The listing builds one solid part. Answer for the finished solid, in the listing's coordinates (mm). A direction names the side the tool comes from. Give positions to 0.01 mm unless a question says otherwise; leave off trailing zeros. Write each loop counter-clockwise with the first axis right and the second up, starting at its lowest first coordinate (ties: lowest second). Pieces come first, ordered by that corner, then holes. Notation, with made-up numbers: (-20.5, 11) - (28.5, 11) arc R31 ccw to (28.5, 35) - close; hole circle Ø8 at (76.5, 62). An arc over 180 degrees is marked (long way). Write each question's results on one line, items separated by ' | '. Start each with the question number.
Q1. Flat-ended cylindrical pins translate along their axes: pin 1 Ø5 at (x, y) = (30.78, -3.04) entering from -Z; pin 2 Ø7 at (x, y) = (6, -4.5) entering from -Z. Find the tip coordinate at first contact, or state that the pin passes through.
Q2. Section C-C (z = -14) is taken. Determine the outline of the cut face in (x, y) (3 decimals).
Q3. Section D-D (x = 33.5) is taken. Determine the outline of the cut face in (y, z) (3 decimals), plus the area to 3 significant figures.
Q4. Section A-A (z = -8.5) is taken. Determine the outline of the cut face in (x, y), plus the area to 3 significant figures.
Q5. Section B-B (y = 1) is taken. Determine the outline of the cut face in (x, z).
Q6. Find the intervals of material crossed by probe 1 along X at (y, z) = (2.25, 9); probe 2 along Z at (x, y) = (7, 0); probe 3 along Z at (x, y) = (22.5, -8.5), in increasing order.
Q7. For a pull along X with two mould halves and no side action, classify faces 4 (the face through (11.43, 0, 2.5)), 5 (the face through (35.56, 0, 0)), 6 (the face through (10, -9.392, -1)) as pulls with the +X half, pulls with the -X half, needs draft (parallel to the pull), parting line crosses it, or undercut.
Q8. For faces 1 (the face through (18, 0, -19.473)), 2 (the face through (5, -3, -13.123)), 3 (the face through (18, 0, -13.123)), determine the directions among +Z, -Z, +X, -X, +Y, -Y from which every point of the face is accessible in a straight line to the end or side of a thin tool.
```python
from build123d import *

# Parameters (mm, degrees)
F0_W     = 19.05
F0_H     = 38.1
F0_R     = 3.175
F1_DEPTH = 35.56
F2_R     = 3.175
F3_DEPTH = 6.35
F4_W     = 12.7
F4_H     = 31.75
F5_DEPTH = 35.56


with BuildPart() as f1:
    # F0 (on Right) → F1 (new body)
    with BuildSketch(Plane.YZ):
        with Locations((0.13327, -0.423332)):
            Rectangle(F0_W, F0_H)
        with Locations((0.13327, 5.926668)):
            Circle(F0_R, mode=Mode.SUBTRACT)
    extrude(amount=F1_DEPTH)

    # F2 (on face) → F3 (cut)
    with BuildSketch(Plane(origin=(0, 0, -19.473332), x_dir=(1, 0, 0), z_dir=(0, 0, -1))):
        with Locations((4.7752, 3.04173)):
            Circle(F2_R)
        with Locations((30.7848, 3.04173)):
            Circle(F2_R)
    extrude(amount=-F3_DEPTH, mode=Mode.SUBTRACT)

    # F4 (on face) → F5 (cut)
    with BuildSketch(Plane.XZ.offset(9.39173)):
        with Locations((17.78, 2.751668)):
            Rectangle(F4_W, F4_H)
    extrude(amount=-F5_DEPTH, mode=Mode.SUBTRACT)


solid = f1.part
```
Answers below:
1) pin 1: stops at z = -13.12 | pin 2: stops at z = -19.47
2) outline: (0, -9.392) - (35.56, -9.392) - (35.56, 9.658) - (0, 9.658) - close; hole circle Ø6.35 at (4.775, -3.042); hole circle Ø6.35 at (30.785, -3.042)
3) outline: (-9.392, -19.473) - (-4.687, -19.473) - (-4.687, -13.123) - (-1.396, -13.123) - (-1.396, -19.473) - (9.658, -19.473) - (9.658, 18.627) - (-9.392, 18.627) - close; hole circle Ø6.35 at (0.133, 5.927) | area: 673 mm2
4) outline: (0, -9.39) - (11.43, -9.39) - (11.43, 9.66) - (0, 9.66) - close; (24.13, -9.39) - (35.56, -9.39) - (35.56, 9.66) - (24.13, 9.66) - close | area: 435 mm2
5) outline: (0, -19.47) - (35.56, -19.47) - (35.56, 2.87) - (24.13, 2.87) - (24.13, -13.12) - (11.43, -13.12) - (11.43, 2.87) - (0, 2.87) - close; (0, 8.98) - (11.43, 8.98) - (11.43, 18.63) - (0, 18.63) - close; (24.13, 8.98) - (35.56, 8.98) - (35.56, 18.63) - (24.13, 18.63) - close
6) probe 1: x = 0 to 11.43, 24.13 to 35.56 | probe 2: z = -19.47 to 2.75, 9.1 to 18.63 | probe 3: z = -19.47 to -13.12
7) face 4: undercut | face 5: pulls with the +X half | face 6: needs draft
8) face 1: -Z, +X, -X, +Y, -Y | face 2: -Z | face 3: +Z, +Y, -Y
